```python
from build123d import *

# Parameters (mm, degrees)
SKETCH1_R           = 4
BOSS_EXTRUDE1_DEPTH = 8
FILLET1_R           = 1


with BuildPart() as part:
    # Sketch1 → Boss-Extrude1 (new body)
    with BuildSketch(Plane.XY):
        with BuildLine():
            Line((0, 10), (0, 25))
            ThreePointArc((0, 25), (25, 0), (0, -25))
            ThreePointArc((0, -25), (-17.5, -7.5), (0, 10))
        make_face()
        with Locations((0, -7.5)):
            Circle(SKETCH1_R, mode=Mode.SUBTRACT)
    extrude(amount=BOSS_EXTRUDE1_DEPTH)

    # Fillet1
    fillet1_edges = [part.edges().sort_by_distance(p)[0] for p in [
        (0, 10, 4),
        (0, 25, 4),
    ]]
    fillet(fillet1_edges, radius=FILLET1_R)


solid = part.part
```
Can you work these out from the model? Positions are in its coordinate system, mm. Coordinates: 2 decimals unless noted, no trailing zeros. Loops run counter-clockwise (first coordinate to the right, second up) from the corner with the lowest first, then second, coordinate; pieces in that order, holes last. Notation, with made-up numbers: M 70,-32 L 101,-32 A33 ccw 101,0 Z; hole C -5,61.25 d9. An arc over 180 degrees is marked long. Put each result on its own line as item: value. Start each with the question number.
(1) I need wall thicknesses on probe 1 along X at (y, z) = (-4, 1.5); probe 2 along X at (y, z) = (-4.5, 4.25); probe 3 along X at (y, z) = (19, 0.75). Which ranges of each line are inside material? Lowest first, please.
(2) Imagine slicing it at C-C on y = 14. List the corners of the cut face in (x, z) for me, and give its area (3 significant figures).
(3) Imagine slicing it at D-D on x = 15. List the corners of the cut face in (y, z) for me, and give its area (3 significant figures).
(4) Imagine slicing it at A-A on x = -3. List the corners of the cut face in (y, z) for me.
(5) Imagine slicing it at B-B on z = 1.5. List the corners of the cut face in (x, y) for me.
(6) We'd pull the mould along X, two halves only. Please class faces 1 (the face through (0, 17, 4)), 2 (the face through (3.815, -6.299, 3.944)), 3 (the face through (4, 0, 0)): +X half, -X half, draft (parallel to the pull), parting line (faces both ways), or undercut.
(7) Will this pin go through, and if not, where does the flat tip stop? pin 1 Ø1 at (x, z) = (-2, 2) entering from +Y.
Worked answers:
1. probe 1: x = -17.15 to -1.94, 1.94 to 24.68
1. probe 2: x = -17.24 to -2.65, 2.65 to 24.59
1. probe 3: x = 0 to 16.25
2. outline: M 0,0 L 20.71,0 L 20.71,8 L 0,8 Z
2. area: 166 mm2
3. outline: M -20,0 L 20,0 L 20,8 L -20,8 Z
3. area: 320 mm2
4. outline: M -24.74,0 L -10.15,0 L -10.15,8 L -24.74,8 Z; M -4.85,0 L 9.74,0 L 9.74,8 L -4.85,8 Z
5. outline: M -0.95,9.97 A17.5 ccw 0,-25 A25 ccw 1.04,24.98 A1 ccw 0,23.98 L 0,10.97 A1 cw Z; hole C 0,-7.5 d8
6. face 1: -X half
6. face 2: undercut
6. face 3: draft
7. pin 1: stops at y = 9.94
